Autodesk Inventor part; units mm, degrees
ref_plane "PLANE RH" through (457.2, 0, 0) normal (1, 0, 0) x (0, 1, 0)
ref_plane "PLANE LH" through (-457.2, 0, 0) normal (1, 0, 0) x (0, 1, 0)
ref_plane "PLANE BOT" through (0, 0, -203.2) normal (0, 0, 1) x (1, 0, 0)
ref_plane "PLANE IN" through (0, 0, 0) normal (0, 1, 0) x (-1, 0, 0)
ref_plane "PLANE OUT" through (0, 1219.2, 0) normal (0, 1, 0) x (-1, 0, 0)
ref_plane "PLANE CTR" through (0, 0, 0) normal (1, 0, 0) x (0, 1, 0)
ref_plane "PLANE RH" through (457.2, 0, 0) normal (1, 0, 0) x (0, 1, 0)
ref_plane "PLANE LH" through (-457.2, 0, 0) normal (1, 0, 0) x (0, 1, 0)
ref_plane "PLANE TOP" through (0, 0, 0) normal (0, 0, 1) x (1, 0, 0)
ref_plane "PLANE BOT" through (0, 0, -203.2) normal (0, 0, 1) x (1, 0, 0)
ref_plane "PLANE HANDLE RH" through (558.8, 0, 0) normal (1, 0, 0) x (0, 1, 0)
ref_plane "PLANE HANDLE LH" through (-558.8, 0, 0) normal (1, 0, 0) x (0, 1, 0)
ref_plane "PLANE HANDLE IN" through (0, 63.5, 0) normal (0, 1, 0) x (-1, 0, 0)
ref_plane "PLANE HANDLE OUT" through (0, 1155.7, 0) normal (0, 1, 0) x (-1, 0, 0)
ref_plane "PLANE HANDLE TOP" through (0, 0, -63.5) normal (0, 0, 1) x (1, 0, 0)
sketch "SKETCH BODY" plane through (0, 0, 0) normal (0, 0, 1) x (1, 0, 0)
  line L0 (-457.2, 0) -> (457.2, 0)
  line L1 (457.2, 0) -> (457.2, 1219.2)
  line L2 (457.2, 1219.2) -> (-457.2, 1219.2)
  line L3 (-457.2, 1219.2) -> (-457.2, 0)
  line L4 (-640.08, 0) -> (640.08, 0)
  line L5 (-640.08, 1219.2) -> (640.08, 1219.2)
  line L6 (457.2, 3657.6) -> (457.2, -609.6)
  line L7 (-457.2, 3657.6) -> (-457.2, -609.6)
extrude "EXT BODY" add sketch "SKETCH BODY" against normal blind 203.2
sketch "SKETCH HANDLE DIA" plane through (457.2, 0, 0) normal (1, 0, 0) x (0, 1, 0)
  line L0 (45.72, -63.5) -> (81.28, -63.5)
  line L1 (63.5, -45.72) -> (63.5, -81.28)
  circle A0 centre (63.5, -63.5) radius 12.7
  dimension "d79" = 25.4
sketch "SKETCH HANDLE PATH" plane through (0, 0, -63.5) normal (0, 0, 1) x (1, 0, 0)
  line L0 (558.8, 3568.7) -> (558.8, -520.7)
  line L1 (457.2, 3568.7) -> (457.2, -520.7)
  line L2 (436.88, 63.5) -> (579.12, 63.5)
  line L3 (436.88, 1155.7) -> (579.12, 1155.7)
  line L4 (457.2, 63.5) -> (558.8, 63.5)
  line L5 (558.8, 63.5) -> (558.8, 1155.7)
  line L6 (558.8, 1155.7) -> (457.2, 1155.7)
  line L7 (457.2, 1155.7) -> (457.2, 63.5) construction
sweep "SWP HANDLE" add profiles "SKETCH HANDLE DIA" path "SKETCH HANDLE PATH" path curves L4 L5 L6
mirror "MIR HANDLE" about plane through (0, 0, 0) normal (1, 0, 0)
equation "\"d76\" = HEIGHT"
equation "\"PLANE_OUT\" = LENGTH"
equation "\"PLANE_RH\" = 0.5 * WIDTH"
equation "\"PLANE_LH\" = -0.5 * WIDTH"
equation "\"PLANE_BOT\" = -HEIGHT"
equation "\"PLANE_HANDLE_RH\" = HANDLE_OFFSET_CTR"
equation "\"PLANE_HANDLE_LH\" = -HANDLE_OFFSET_CTR"
equation "\"PLANE_HANDLE_IN\" = HANDLE_OFFSET_END"
equation "\"PLANE_HANDLE_OUT\" = LENGTH - HANDLE_OFFSET_END"
equation "\"PLANE_HANDLE_TOP\" = -HANDLE_OFFSET_TOP"
equation "\"LENGTH\" = 1219.2"
equation "\"WIDTH\" = 914.4"
equation "\"HEIGHT\" = 203.2"
equation "\"HANDLE_GAP\" = 101.6"
equation "\"HANDLE_OFFSET_CTR\" = 0.5 * WIDTH + HANDLE_GAP"
equation "\"HANDLE_OFFSET_END\" = 63.5"
equation "\"HANDLE_OFFSET_TOP\" = 63.5"
properties part number "Blog Part"
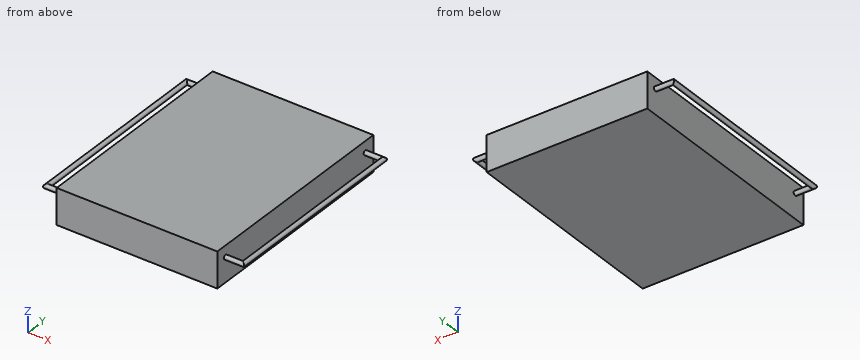
The listing builds one solid part. Answer for the finished solid, in the listing's coordinates (mm). Give positions to 0.01 mm unless a question says otherwise; leave off trailing zeros. Order: outer loops, then holes, each group sorted by start corner. A loop starts at its lowest first (then second) coordinate and runs counter-clockwise, first axis right, second up. Notation, with made-up numbers: (-7, 44) -> (43, 44) arc R30 cw to (43, 81) -> close; hole circle Ø1 at (53, 41.25). An arc over 180 degrees is marked (long way). Write each question's results on one line, items separated by ' | '.
Q1. Each of these flat-tipped pins is pushed along its axis until it touches: P1, Ø4, axis at y = 136, z = -23.5, coming from the -X side; P2, Ø4, axis at y = 792.5, z = -26.5, coming from the +X side. Where does it stop, or does it pass through?
Checked values:
P1: stops at x = -457.2 | P2: stops at x = 457.2
Q2. The part is cut by section B-B, the plane x = 489. Give the vertices of the cut face in (y, z).
Checked values:
outline: circle Ø25.4 at (63.5, -63.5); circle Ø25.4 at (1155.7, -63.5)
Q3. The part is cut by section A-A, the plane y = 156. Give the vertices of the cut face in (x, z), and give its area (3 significant figures).
Checked values:
outline: circle Ø25.4 at (-558.8, -63.5); (-457.2, -203.2) -> (457.2, -203.2) -> (457.2, 0) -> (-457.2, 0) -> close; circle Ø25.4 at (558.8, -63.5) | area: 187,000 mm^2
Q4. Straight lines are drawn through the part: probe 1 along X at (y, z) = (784, -66); probe 2 along X at (y, z) = (1116.5, -143). For each, find the intervals that lie inside material, in ascending order. Write a range as from..to.
Checked values:
probe 1: x = -571.25..-546.35, -457.2..457.2, 546.35..571.25 | probe 2: x = -457.2..457.2
